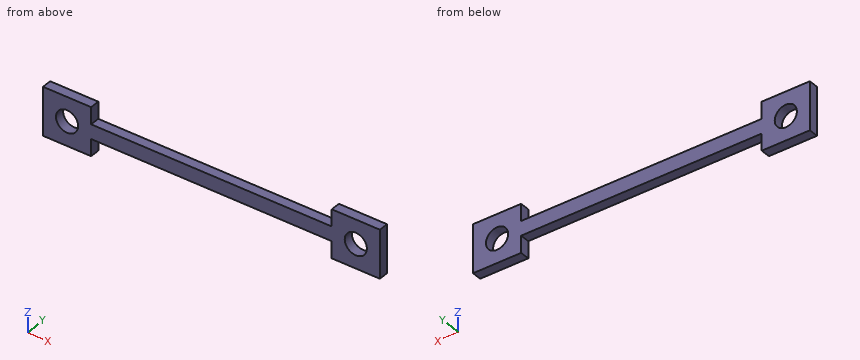
```python
from build123d import *

# Parameters (mm, degrees)
BOSS_EXTRUDE1_DEPTH          = 0.635
F_97_0_0059_DIAMETER_HOLE1_D = 2.921


with BuildPart() as part:
    # Sketch1 → Boss-Extrude1 (new, symmetric)
    with BuildSketch(Plane(origin=(0, 0, 0), x_dir=(1, 0, 0), z_dir=(0, 1, 0))):
        Polygon((-41.424046485, -10.283259465), (-41.424046485, -12.505759465), (-47.774046485, -12.505759465), (-47.774046485, -6.155759465), (-41.424046485, -6.155759465), (-41.424046485, -8.378259465), (-9.674046485, -8.378259465), (-9.674046485, -6.155759465), (-3.324046485, -6.155759465), (-3.324046485, -12.505759465), (-9.674046485, -12.505759465), (-9.674046485, -10.283259465), align=None)
    extrude(amount=BOSS_EXTRUDE1_DEPTH, both=True)

    # #97 (0.0059) Diameter Hole1 (through all)
    with Locations(Plane(origin=(0, 0.635, 0), x_dir=(-1, 0, 0), z_dir=(0, 1, 0))):
        with Locations((44.599046485, 9.330759465)):
            f_97_0_0059_diameter_hole1 = Hole(F_97_0_0059_DIAMETER_HOLE1_D / 2)

    # Mirror1: #97 (0.0059) Diameter Hole1 across plane
    add(f_97_0_0059_diameter_hole1.mirror(Plane(origin=(-25.549046485, 0, 0), x_dir=(0, 0, 1), z_dir=(1, 0, 0))), mode=Mode.SUBTRACT)


solid = part.part
```
CAD build for the part. Positions are in the model's coordinates, mm. Give positions to 0.01 mm unless a question says otherwise; leave off trailing zeros. Loops run counter-clockwise (first coordinate to the right, second up) from the corner with the lowest first, then second, coordinate; pieces in that order, holes last. Notation, with made-up numbers: (77.25, 7.25) - (113.25, 7.25) arc R24 ccw to (113.25, 27.25) - close; hole circle Ø10 at (19, 12.25). An arc over 180 degrees is marked (long way). Put each result on its own line as item: value.
Q1. Slice it at A-A (z = 7.5). Give the cut face in (x, y) (3 decimals).
Filled in:
outline: (-47.774, -0.635) - (-41.424, -0.635) - (-41.424, 0.635) - (-47.774, 0.635) - close; (-9.674, -0.635) - (-3.324, -0.635) - (-3.324, 0.635) - (-9.674, 0.635) - close
Q2. Slice it at B-B (y = 0.05). Give the cut face in (x, z), plus the area to 3 significant figures.
Filled in:
outline: (-47.77, 6.16) - (-41.42, 6.16) - (-41.42, 8.38) - (-9.67, 8.38) - (-9.67, 6.16) - (-3.32, 6.16) - (-3.32, 12.51) - (-9.67, 12.51) - (-9.67, 10.28) - (-41.42, 10.28) - (-41.42, 12.51) - (-47.77, 12.51) - close; hole circle Ø2.92 at (-44.6, 9.33); hole circle Ø2.92 at (-6.5, 9.33)
area: 128 mm²
Q3. Probe line 1 along X through (y, z) = (0.2, 9.25); line 2 along X through (y, z) = (0.5, 11.5); line 3 along X through (y, z) = (0.25, 9.75). List the from-to ranges inside material, lowest first.
Filled in:
line 1: x = -47.77 to -46.06, -43.14 to -7.96, -5.04 to -3.32
line 2: x = -47.77 to -41.42, -9.67 to -3.32
line 3: x = -47.77 to -46, -43.2 to -7.9, -5.1 to -3.32
Q4. Slice it at C-C (x = -10.5). Give the cut face in (y, z) (3 decimals).
Filled in:
outline: (-0.635, 8.378) - (0.635, 8.378) - (0.635, 10.283) - (-0.635, 10.283) - close
Q5. Flat gauge pin, fed straight in: pin 1 (0.6 mm diameter, centred on x = -29.5, y = 0.5, fed in from -Z). Where does the tip first touch, or does it go through?
Filled in:
pin 1: stops at z = 8.38
